from build123d import *

# Parameters (mm, degrees)
F1_DEPTH = 18
F3_DEPTH = 200
F4_R     = 15


with BuildPart() as f1:
    # F0 (on Front) → F1 (new body)
    with BuildSketch(Plane.XZ):
        with BuildLine():
            Line((0, -380), (0, 0))
            Line((0, 0), (-200, 0))
            Line((-200, 0), (-200, -380))
            Line((-200, -380), (-183.066239, -380))
            ThreePointArc((-183.066239, -380), (-100, -370), (-16.933761, -380))
            Line((-16.933761, -380), (0, -380))
        make_face()
    extrude(amount=F1_DEPTH)

    # F2 (on face) → F3 (cut, through all)
    with BuildSketch(Plane(origin=(-200, 0, 0), x_dir=(0, -1, 0), z_dir=(-1, 0, 0))):
        Polygon((18, -49.454594), (18, 0), (0, 0), align=None)
    extrude(amount=-F3_DEPTH, mode=Mode.SUBTRACT)

    # F4
    f4_edges = [f1.edges().sort_by_distance(p)[0] for p in [
        (-200, -9, -380),
        (0, -9, -380),
    ]]
    fillet(f4_edges, radius=F4_R)


solid = f1.part
Input: part model. Units: mm. Frame: model coordinates. Coordinates: 2 decimals unless noted, no trailing zeros. Loops run counter-clockwise (first coordinate to the right, second up) from the corner with the lowest first, then second, coordinate; pieces in that order, holes last.
(1) Section B-B on x = -96. Return the cut outline in (y, z).
(2) First-contact query: pin 1 Ø6 at (x, z) = (-36.5, -253) entering from +Y; pin 2 Ø5 at (x, y) = (-142.5, -10) entering from -Z. Flat tips, straight axial feed; report the tip coordinate or a pass-through.
(3) Section A-A on y = -13. Return the cut outline in (x, z), then the cut area to 3 significant figures.
(4) Material intervals for probe 1 along Y at (x, z) = (-178.5, -32.5); probe 2 along Y at (x, z) = (-150, -30.5), sorted ascending.
(5) Section C-C on z = -42.5. Return the cut outline in (x, y), then the cut area to 3 significant figures.
(6) Pull-direction query (Z, two-part tool) for faces 1 (the face through (-101.4, -8.874, -24.381)), 2 (the face through (-101, -9, -370)), 3 (the face through (-200, -9, -180)); classes: released by +Z, released by -Z, zero draft, split by the parting line, or undercut.
Data:
1. outline: (-18, -370.02) - (0, -370.02) - (0, 0) - (-18, -49.45) - close
2. pin 1: stops at y = 0
2. pin 2: stops at z = -372.9
3. outline: (-200, -365) arc R15 ccw to (-185, -380) - (-183.07, -380) arc R350 cw to (-16.93, -380) - (-15, -380) arc R15 ccw to (0, -365) - (0, -35.72) - (-200, -35.72) - close
3. area: 67,600 mm2
4. probe 1: y = -11.83 to 0
4. probe 2: y = -11.1 to 0
5. outline: (-200, -15.47) - (0, -15.47) - (0, 0) - (-200, 0) - close
5. area: 3,090 mm2
6. face 1: released by +Z
6. face 2: released by -Z
6. face 3: zero draft
